```python
from build123d import *

# Parameters (mm, degrees)
BOSS_EXTRUDE1_DEPTH = 500
SKETCH4_R           = 3
CUT_EXTRUDE1_DEPTH  = 4.5
SKETCH6_R           = 1.75
CUT_EXTRUDE2_DEPTH  = 501.086492519
LPATTERN1_COUNT     = 13
LPATTERN1_PITCH     = 40


with BuildPart() as part:
    # Sketch1 → Boss-Extrude1 (new body)
    with BuildSketch(Plane.XY):
        Polygon((6.7, 5), (-6.7, 5), (-7.5, 4.2), (-7.5, 3.4), (-6.7, 2.6), (-5.9, 2.6), (-5.9, 1.6), (-6.7, 1.6), (-7.5, 0.8), (-7.5, -4.2), (-6.7, -5), (6.7, -5), (7.5, -4.2), (7.5, 0.8), (6.7, 1.6), (5.9, 1.6), (5.9, 2.6), (6.7, 2.6), (7.5, 3.4), (7.5, 4.2), align=None)
    extrude(amount=BOSS_EXTRUDE1_DEPTH)

    # Sketch4 → Cut-Extrude1 (cut)
    with BuildSketch(Plane(origin=(0, 5, 0), x_dir=(1, 0, 0), z_dir=(0, 1, 0))):
        with Locations(Location((0, -10, 0), (0, 0, 270))):
            Circle(SKETCH4_R)
    cut_extrude1 = extrude(amount=-CUT_EXTRUDE1_DEPTH, mode=Mode.SUBTRACT)

    # Sketch6 → Cut-Extrude2 (cut, through all)
    with BuildSketch(Plane(origin=(0, 0.5, 0), x_dir=(1, 0, 0), z_dir=(0, 1, 0))):
        with Locations(Location((0, -10, 0), (0, 0, 270))):
            Circle(SKETCH6_R)
    cut_extrude2 = extrude(amount=-CUT_EXTRUDE2_DEPTH, mode=Mode.SUBTRACT)

    # LPattern1: Cut-Extrude1, Cut-Extrude2 ×13
    with Locations(*[(0, 0, i * LPATTERN1_PITCH) for i in range(1, LPATTERN1_COUNT)]):
        add(cut_extrude1, mode=Mode.SUBTRACT)
        add(cut_extrude2, mode=Mode.SUBTRACT)


solid = part.part
```
Input: part model. Units: mm. Frame: model coordinates. Round coordinates to 2 decimals unless told otherwise and drop trailing zeros. Loops run counter-clockwise (first coordinate to the right, second up) from the corner with the lowest first, then second, coordinate; pieces in that order, holes last. Notation, with made-up numbers: (13, 7) -> (53, 7) arc R28 cw to (53, 26) -> close; hole circle Ø1 at (-19, 77). An arc over 180 degrees is marked (long way). Write each question's results on one line, items separated by ' | '.
1. First-contact query: P1, Ø3, axis at x = -1, z = 491, coming from the +Y side. Flat tip, straight axial feed; report the tip coordinate or a pass-through.
Geometry results:
P1: y = 0.5
2. Ray query, line 1 (Y direction, x = -6, z = 212.5); line 2 (X direction, y = -3.9, z = 490); line 3 (Y direction, x = 6.75, z = 45). Return the intervals inside material, ascending. Write a range as from..to.
Geometry results:
line 1: -5..1.6, 2.6..5 | line 2: -7.5..-1.75, 1.75..7.5 | line 3: -4.95..1.55, 2.65..4.95
3. Section A-A (z = 180). Return loops of the section in (x, y).
Geometry results:
outline: (-7.5, -4.2) -> (-6.7, -5) -> (6.7, -5) -> (7.5, -4.2) -> (7.5, 0.8) -> (6.7, 1.6) -> (5.9, 1.6) -> (5.9, 2.6) -> (6.7, 2.6) -> (7.5, 3.4) -> (7.5, 4.2) -> (6.7, 5) -> (-6.7, 5) -> (-7.5, 4.2) -> (-7.5, 3.4) -> (-6.7, 2.6) -> (-5.9, 2.6) -> (-5.9, 1.6) -> (-6.7, 1.6) -> (-7.5, 0.8) -> close
